```python
from build123d import *

# Parameters (mm, degrees)
SKETCH_2_R      = 1.65
SKETCH_2_R_2    = 4.9
SKETCH_2_R_3    = 2.5
SKETCH_2_R_4    = 2
EXTRUDE_1_DEPTH = 3


with BuildPart() as part:
    # Sketch 2 → Extrude 1 (new body)
    with BuildSketch(Plane.XY):
        Polygon((40, 0), (260, 0), (260, 90), (300, 90), (300, 220), (260, 220), (260, 310), (300, 310), (300, 340), (252.5, 340), (252.5, 330), (47.5, 330), (47.5, 340), (0, 340), (0, 310), (40, 310), (40, 220), (0, 220), (0, 90), (40, 90), align=None)
        with Locations((50.85, 273)):
            Circle(SKETCH_2_R, mode=Mode.SUBTRACT)
        with Locations((64.85, 273)):
            Circle(SKETCH_2_R, mode=Mode.SUBTRACT)
        with Locations(Location((64.85, 257, 0), (0, 0, 180))):
            Circle(SKETCH_2_R, mode=Mode.SUBTRACT)
        with Locations(Location((50.85, 257, 0), (0, 0, 180))):
            Circle(SKETCH_2_R, mode=Mode.SUBTRACT)
        with Locations((57.8, 265)):
            Circle(SKETCH_2_R_2, mode=Mode.SUBTRACT)
        with Locations((235.15, 257)):
            Circle(SKETCH_2_R, mode=Mode.SUBTRACT)
        with Locations((249.15, 257)):
            Circle(SKETCH_2_R, mode=Mode.SUBTRACT)
        with Locations(Location((242.2, 265, 0), (0, 0, 180))):
            Circle(SKETCH_2_R_2, mode=Mode.SUBTRACT)
        with Locations(Location((235.15, 273, 0), (0, 0, 180))):
            Circle(SKETCH_2_R, mode=Mode.SUBTRACT)
        with Locations(Location((249.15, 273, 0), (0, 0, 180))):
            Circle(SKETCH_2_R, mode=Mode.SUBTRACT)
        with Locations(Location((249.15, 53, 0), (0, 0, 180))):
            Circle(SKETCH_2_R, mode=Mode.SUBTRACT)
        with Locations(Location((235.15, 53, 0), (0, 0, 180))):
            Circle(SKETCH_2_R, mode=Mode.SUBTRACT)
        with Locations((249.15, 37)):
            Circle(SKETCH_2_R, mode=Mode.SUBTRACT)
        with Locations((242.2, 45)):
            Circle(SKETCH_2_R_2, mode=Mode.SUBTRACT)
        with Locations((235.15, 37)):
            Circle(SKETCH_2_R, mode=Mode.SUBTRACT)
        with Locations((50.85, 53)):
            Circle(SKETCH_2_R, mode=Mode.SUBTRACT)
        with Locations((64.85, 53)):
            Circle(SKETCH_2_R, mode=Mode.SUBTRACT)
        with Locations(Location((64.85, 37, 0), (0, 0, 180))):
            Circle(SKETCH_2_R, mode=Mode.SUBTRACT)
        with Locations(Location((57.8, 45, 0), (0, 0, 180))):
            Circle(SKETCH_2_R_2, mode=Mode.SUBTRACT)
        with Locations(Location((50.85, 37, 0), (0, 0, 180))):
            Circle(SKETCH_2_R, mode=Mode.SUBTRACT)
        with Locations((23.5, 333.5)):
            Circle(SKETCH_2_R_3, mode=Mode.SUBTRACT)
        with Locations((23.5, 316.5)):
            Circle(SKETCH_2_R_3, mode=Mode.SUBTRACT)
        with Locations(Location((276.5, 316.5, 0), (0, 0, 180))):
            Circle(SKETCH_2_R_3, mode=Mode.SUBTRACT)
        with Locations(Location((276.5, 333.5, 0), (0, 0, 180))):
            Circle(SKETCH_2_R_3, mode=Mode.SUBTRACT)
        with Locations((23.5, 119.5)):
            Circle(SKETCH_2_R_3, mode=Mode.SUBTRACT)
        with Locations((23.5, 102.5)):
            Circle(SKETCH_2_R_3, mode=Mode.SUBTRACT)
        with Locations(Location((276.5, 102.5, 0), (0, 0, 180))):
            Circle(SKETCH_2_R_3, mode=Mode.SUBTRACT)
        with Locations(Location((276.5, 119.5, 0), (0, 0, 180))):
            Circle(SKETCH_2_R_3, mode=Mode.SUBTRACT)
        with Locations((179.787668085, 215.90015868)):
            Circle(SKETCH_2_R_4, mode=Mode.SUBTRACT)
        with Locations((189.787668085, 215.90015868)):
            Circle(SKETCH_2_R_4, mode=Mode.SUBTRACT)
        with Locations((179.787668085, 163.90015868)):
            Circle(SKETCH_2_R_4, mode=Mode.SUBTRACT)
        with Locations((189.787668085, 163.90015868)):
            Circle(SKETCH_2_R_4, mode=Mode.SUBTRACT)
    extrude(amount=EXTRUDE_1_DEPTH)


solid = part.part
```
For this review, take the finished solid that the model builds, in its own axes (mm). Coordinates: 2 decimals unless noted, no trailing zeros. Write each loop counter-clockwise with the first axis right and the second up, starting at its lowest first coordinate (ties: lowest second). Pieces come first, ordered by that corner, then holes. Notation, with made-up numbers: (58.25, 32.5) -> (116.25, 32.5) arc R16 cw to (116.25, 60.5) -> close; hole circle Ø2 at (80, 54.5). An arc over 180 degrees is marked (long way). Put each result on its own line as item: value.
Q1. The part is to be moulded in two halves that separate along X. For faces 1 (the flat face through (148, 172, 0)), 2 (the cylindrical face through (237.526, 263.528, 1.479)), say which applies: +X half, -X half, draft (parallel to the pull), parting line (faces both ways), or undercut.
From the geometry:
face 1: draft
face 2: undercut
Q2. Take a section at B-B, the plane y = 265. State the section outline as (x, z) points.
From the geometry:
outline: (40, 0) -> (52.9, 0) -> (52.9, 3) -> (40, 3) -> close; (62.7, 0) -> (237.3, 0) -> (237.3, 3) -> (62.7, 3) -> close; (247.1, 0) -> (260, 0) -> (260, 3) -> (247.1, 3) -> close
Q3. Take a section at A-A, the plane x = 242.2. State the section outline as (y, z) points, then the cut area to 3 significant figures.
From the geometry:
outline: (0, 0) -> (40.1, 0) -> (40.1, 3) -> (0, 3) -> close; (49.9, 0) -> (260.1, 0) -> (260.1, 3) -> (49.9, 3) -> close; (269.9, 0) -> (330, 0) -> (330, 3) -> (269.9, 3) -> close
area: 931 mm2
Q4. Take a section at C-C, the plane x = 72.5. State the section outline as (y, z) points.
From the geometry:
outline: (0, 0) -> (330, 0) -> (330, 3) -> (0, 3) -> close
Q5. Wall thickness on L1, parallel to Y at x = 23.5, z = 1.2; L2, parallel to Y at x = 235.15, z = 2.3; L3, parallel to Y at x = 242.2, z = 1.35: over which ranges is each line inside the solid? List them lowest first.
From the geometry:
L1: y = 90 to 100, 105 to 117, 122 to 220, 310 to 314, 319 to 331, 336 to 340
L2: y = 0 to 35.35, 38.65 to 51.35, 54.65 to 255.35, 258.65 to 271.35, 274.65 to 330
L3: y = 0 to 40.1, 49.9 to 260.1, 269.9 to 330
Q6. Take a section at D-D, the plane z = 2.4. Count the separate pieces of the cut face and the enclosed holes in it, then the cut area to 3 significant figures.
From the geometry:
separate pieces: 1
enclosed holes: 32
area: 84,900 mm2
Q7. Clearance check with flat-ended pins moving along their axes: pin 1 Ø0.9 at (y, z) = (257.5, 1) entering from +X; pin 2 Ø2 at (x, y) = (235.15, 257) entering from -Z; pin 3 Ø8 at (x, y) = (23.5, 333.5) entering from -Z. State where each tip first meets the part, or that it passes through.
From the geometry:
pin 1: stops at x = 260
pin 2: passes through
pin 3: stops at z = 0
